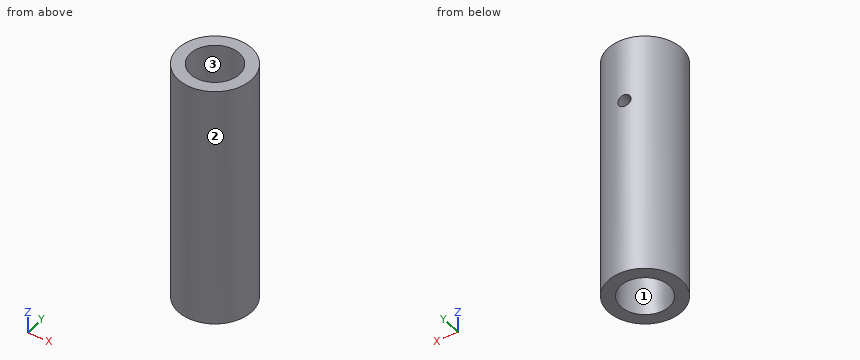
```python
from build123d import *

# Parameters (mm, degrees)
SKETCH1_R           = 9.525
BOSS_EXTRUDE1_DEPTH = 63.5
SKETCH3_R           = 6.35
CUT_EXTRUDE2_DEPTH  = 48.26


# Read off the part's stored shape, not the designer's step: 1/8 (0.125) Diameter Hole1
with BuildPart() as part:
    # Sketch1 → Boss-Extrude1 (new body)
    with BuildSketch(Plane.XY):
        Circle(SKETCH1_R)
    extrude(amount=BOSS_EXTRUDE1_DEPTH)

    # Sketch3 → Cut-Extrude2 (cut)
    with BuildSketch(Plane.XY.offset(63.5)):
        Circle(SKETCH3_R)
    extrude(amount=-CUT_EXTRUDE2_DEPTH, mode=Mode.SUBTRACT)

    # 1/8 (0.125) Diameter Hole1 outline → 1/8 (0.125) Diameter Hole1 (revolve, cut)
    with BuildSketch(Plane(origin=(0, 0, 46.736), x_dir=(0.99452895474108, 0.10446127599074502, 0), z_dir=(0, 0, -1))):
        Polygon((1.5875, -9.525019471), (1.5875, -6.35), (1.346904209, -6.205435464), (0, -6.205435464), (0, -9.525019471), align=None)
    revolve(axis=Axis((0, 0, 46.736), (0.10446127599074502, -0.99452895474108, 0)), mode=Mode.SUBTRACT)

    # Sketch11 → 1/4 NPT Tapped Hole1 (revolve, cut)
    with BuildSketch(Plane.YZ):
        Polygon((0, 0), (0, 19.852347279), (5.5626, 16.51), (5.5626, 12.7), (5.943684593, 12.7), (6.3239396, 0), align=None)
    revolve(axis=Axis((0, 0, -6.35), (0, 0, 1)), mode=Mode.SUBTRACT)


solid = part.part
```
CAD build for the part. Positions are in the model's coordinates, mm. Face numbers are marked on the shaded views. Round coordinates to 2 decimals unless told otherwise and drop trailing zeros. Loops run counter-clockwise (first coordinate to the right, second up) from the corner with the lowest first, then second, coordinate; pieces in that order, holes last. Notation, with made-up numbers: (26, 61.5) - (47, 61.5) arc R26 ccw to (47, 89.5) - close; hole circle Ø11 at (-15.5, 67). An arc over 180 degrees is marked (long way). Return JSON: item names as keys, results as strings. Group by question number.
Q1. Band-saw the part on B-B on x = 0. Give the number of separate pieces and of enclosed holes in the cut face, plus the area to 3 significant figures.
Q2. Band-saw the part on A-A on z = 20. Give the cut face in (x, y) (3 decimals), plus the area to 3 significant figures.
Q3. Flat gauge pins, fed straight in: pin 1 Ø6 at (y, z) = (-6, 53.5) entering from -X; pin 2 Ø5 at (x, y) = (-0.5, -5.5) entering from +Z; pin 3 Ø6 at (y, z) = (3.5, 44) entering from +X; pin 4 Ø1.5 at (y, z) = (-6.5, 33.5) entering from -X. Where does each tip first touch, or does it go through?
Q4. Drill centre lines: line 1 along Y through (x, z) = (0, 13.85) (3 decimals); line 2 along Y through (x, z) = (-2.5, 60.5); line 3 along Z through (x, y) = (5.75, 0.75). Where is each one in solid material? Low to high. Write a range as [from, to].
Q5. Two-plate mould, pull along X, no slides. Class the marked faces 1, 2 and 3: +X half, -X half, draft (parallel to the pull), parting line (faces both ways), or undercut.
Solutions:
{
 "1": {"separate pieces": "3", "enclosed holes": "0", "area": "404 mm^2"},
 "2": {"outline": "circle Ø19.05 at (0, 0); hole circle Ø12.7 at (0, 0)", "area": "158 mm^2"},
 "3": {"pin 1": "stops at x = -9.04", "pin 2": "stops at z = 63.5", "pin 3": "stops at x = 9.51", "pin 4": "stops at x = -7.59"},
 "4": {"line 1": "y = [-9.525, -5.563], [5.563, 9.525]", "line 2": "y = [-9.19, -5.84], [5.84, 9.19]", "line 3": "z = [12.7, 15.24]"},
 "5": {"face 1": "undercut", "face 2": "parting line", "face 3": "undercut"}
}
